Build history of the part. All positions in model axes, mm. Face numbers are marked on the shaded views. A direction names the side the tool comes from. Round coordinates to 2 decimals unless told otherwise and drop trailing zeros. Write each loop counter-clockwise with the first axis right and the second up, starting at its lowest first coordinate (ties: lowest second). Pieces come first, ordered by that corner, then holes. Notation, with made-up numbers: M 30,-36.75 L 82,-36.75 A28 cw 82,-15.75 Z; hole C 41,38.5 d8. An arc over 180 degrees is marked long. Use a Markdown table: item, result.
from build123d import *

# Parameters (mm, degrees)
EXTRUDE_3_DEPTH     = 5
SKETCH_1_R          = 9.79888
CUT_EXTRUDE_1_DEPTH = 1.65
SKETCH_1_9_R        = 3.15
SKETCH_3_8_R        = 1.65
SKETCH_3_9_R        = 1.648905
SKETCH_3_9_R_2      = 1.65
CUT_EXTRUDE_2_DEPTH = 5
EXTRUDE_4_DEPTH     = 28
SKETCH_10_R         = 11.19888
CUT_EXTRUDE_3_DEPTH = 3.35


with BuildPart() as part:
    # 草图7 → 凸台-拉伸3 (new body)
    with BuildSketch(Plane.XY):
        with BuildLine():
            Line((14, 14), (-14, 14))
            Line((-14, 14), (-14, 0))
            ThreePointArc((-14, 0), (-12.934313455, -5.357568053), (-9.899494937, -9.899494937))
            Line((-9.899494937, -9.899494937), (-2.121320344, -17.67766953))
            ThreePointArc((-2.121320344, -17.67766953), (0.000404905, -18.556181469), (2.121892965, -17.677096908))
            Line((2.121892965, -17.677096908), (9.899494937, -9.899494937))
            ThreePointArc((9.899494937, -9.899494937), (12.934313455, -5.357568053), (14, 0))
            Line((14, 0), (14, 14))
        make_face()
    extrude(amount=-EXTRUDE_3_DEPTH)

    # 草图1 → 切除-拉伸1 (cut)
    with BuildSketch(Plane.XY):
        Circle(SKETCH_1_R)
    extrude(amount=-CUT_EXTRUDE_1_DEPTH, mode=Mode.SUBTRACT)

    # 切除-放样1: read off the stored shape, not the designer's step
    # 切除-放样1 outline → 切除-放样1 (revolve, cut)
    with BuildSketch(Plane(origin=(10.6066, 10.606603436, 0), x_dir=(1, 0, 0), z_dir=(0, -1, 0))):
        Polygon((0, 0), (0, -1.5), (1.648905, -1.5), (3.15, 0), align=None)
    revolve(axis=Axis((10.6066, 10.606603436, 0), (0, 0, 1)), mode=Mode.SUBTRACT)

    # 切除-放样2: read off the stored shape, not the designer's step
    # 切除-放样2: loft between two sections, ruled curve by curve
    loft_2_from = [
        Edge.make_bspline([(-8.058196468, 12.45812698, 0), (-4.355149378, 7.361319916, 0), (-9.451956443, 3.658272826, 0), (-13.155003532, 8.755079891, 0), (-16.858050622, 13.851886955, 0), (-11.761243557, 17.554934045, 0), (-8.058196468, 12.45812698, 0)], [0, 0, 0, 0, 0.5, 0.5, 0.5, 1, 1, 1, 1], 3, [1, 0.333333333, 0.333333333, 1, 0.333333333, 0.333333333, 1]),
    ]
    loft_2_to = [
        Edge.make_bspline([(-9.518492924, 11.845518562, -1.5), (-7.040662671, 9.669304411, -1.5), (-9.216876823, 7.191474158, -1.5), (-11.694707076, 9.367688309, -1.5), (-14.172537329, 11.543902461, -1.5), (-11.996323177, 14.021732714, -1.5), (-9.518492924, 11.845518562, -1.5)], [0, 0, 0, 0, 0.5, 0.5, 0.5, 1, 1, 1, 1], 3, [1, 0.333333333, 0.333333333, 1, 0.333333333, 0.333333333, 1]),
    ]
    loft_2 = Solid(Shell([*[Face.make_surface_from_curves(loft_2_from[k], loft_2_to[k]) for k in range(1)], Face(Wire(loft_2_from)), Face(Wire(loft_2_to))]))
    add(loft_2, mode=Mode.SUBTRACT)

    # 草图1<9> → 切除-放样3 section 0
    with BuildSketch(Plane.XY):
        with Locations((0, -14.999996564)):
            Circle(SKETCH_1_9_R)
    # 草图3<8> → 切除-放样3 section 1
    with BuildSketch(Plane.XY.offset(-1.5)):
        with Locations((0, -14.999996564)):
            Circle(SKETCH_3_8_R)
    loft(mode=Mode.SUBTRACT)

    # 草图3<9> → 切除-拉伸2 (cut)
    with BuildSketch(Plane.XY.offset(-1.5)):
        with Locations(Location((-10.6066, 10.606603436, 0), (0, 0, 48.708))):
            Circle(SKETCH_3_9_R)
        with Locations((10.6066, 10.606603436)):
            Circle(SKETCH_3_9_R)
        with Locations((0, -14.999996564)):
            Circle(SKETCH_3_9_R_2)
    extrude(amount=-CUT_EXTRUDE_2_DEPTH, mode=Mode.SUBTRACT)

    # 草图9 → 凸台-拉伸4 (add)
    with BuildSketch(Plane(origin=(14, 0, 0), x_dir=(0, 0, -1), z_dir=(1, 0, 0))):
        Polygon((5, 14), (5, 16), (2, 16), (0, 14), align=None)
    extrude(amount=-EXTRUDE_4_DEPTH)

    # 草图10 → 切除-拉伸3 (cut)
    with BuildSketch(Plane(origin=(0, 0, -5), x_dir=(-1, 0, 0), z_dir=(0, 0, -1))):
        Circle(SKETCH_10_R)
    extrude(amount=-CUT_EXTRUDE_3_DEPTH, mode=Mode.SUBTRACT)


solid = part.part
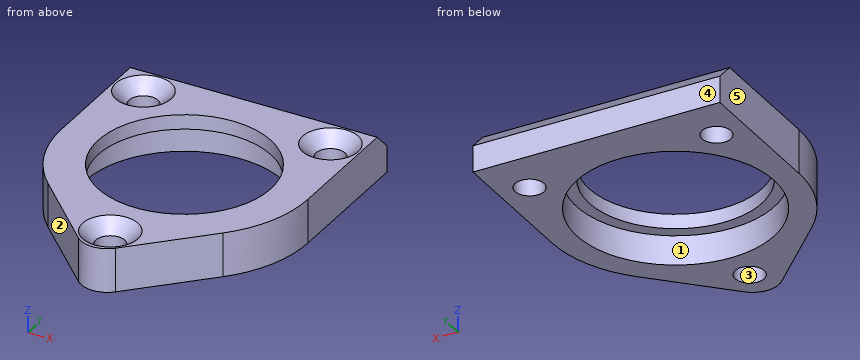
Q1. Two-plate mould, pull along Y, no slides. Class the marked faces 3, 4 and 5: +Y half, -Y half, draft (parallel to the pull), parting line (faces both ways), or undercut.
Response values:
| item | result |
|---|---|
| face 3 | undercut |
| face 4 | +Y half |
| face 5 | draft |
Q2. Drop flat-ended pins along their axis: P1, Ø3, axis at x = 0, y = -15, coming from the +Z side; P2, Ø1.5, axis at y = -12.5, z = -4.5, coming from the -X side. Give the stop position or say it passes through.
Response values:
| item | result |
|---|---|
| P1 | passes through |
| P2 | stops at x = -8.05 |
Q3. Cut at B-B on y = 6. Give the cut face in (x, z).
Response values:
| item | result |
|---|---|
| outline | M -14,-5 L -9.46,-5 L -9.46,-1.65 L -7.75,-1.65 L -7.75,0 L -14,0 Z; M 7.75,-1.65 L 9.46,-1.65 L 9.46,-5 L 14,-5 L 14,0 L 7.75,0 Z |
Q4. Cut at C-C on z = -3.5. Give the cut face in (x, y).
Response values:
| item | result |
|---|---|
| outline | M -14,0 A14 ccw -9.9,-9.9 L -2.12,-17.68 A3 ccw 2.12,-17.68 L 9.9,-9.9 A14 ccw 14,0 L 14,16 L -14,16 Z; hole C -10.61,10.61 d3.3; hole C 0,0 d22.4; hole C 0,-15 d3.3; hole C 10.61,10.61 d3.3 |
Q5. Cut at A-A on x = 0. Give the cut face in (y, z), and give its area (3 significant figures).
Response values:
| item | result |
|---|---|
| outline | M -18.56,-5 L -16.65,-5 L -16.65,-1.5 L -18.15,0 L -18.56,0 Z; M -13.35,-5 L -11.2,-5 L -11.2,-1.65 L -9.8,-1.65 L -9.8,0 L -11.85,0 L -13.35,-1.5 Z; M 9.8,-1.65 L 11.2,-1.65 L 11.2,-5 L 16,-5 L 16,-2 L 14,0 L 9.8,0 Z |
| area | 44.7 mm2 |
Q6. Cut at D-D on x = -4.75. Give the cut face in (y, z), and give its area (3 significant figures).
Response values:
| item | result |
|---|---|
| outline | M -15.05,-5 L -10.14,-5 L -10.14,-1.65 L -8.57,-1.65 L -8.57,0 L -15.05,0 Z; M 8.57,-1.65 L 10.14,-1.65 L 10.14,-5 L 16,-5 L 16,-2 L 14,0 L 8.57,0 Z |
| area | 57.0 mm2 |
Q7. Which spindle directions (+Z, -Z, +X, -X, +Y, -Y) get a long thin tool onto all of the face, cutting with end or side? Do the marked faces 1 and 2. Say none if no direction does.
Response values:
| item | result |
|---|---|
| face 1 | -Z |
| face 2 | +Z, -Z, -X, -Y |
Q8. Drill centre lines: L1, parallel to Y at x = 0, z = -3.15; L2, parallel to Y at x = 0, z = -1; L3, parallel to X at y = 10, z = -4.1. Where is each one in solid material? Low to high.
Response values:
| item | result |
|---|---|
| L1 | y = -18.56 to -16.65, -13.35 to -11.2, 11.2 to 16 |
| L2 | y = -18.56 to -17.15, -12.85 to -9.8, 9.8 to 15 |
| L3 | x = -14 to -12.14, -9.07 to -5.04, 5.04 to 9.07, 12.14 to 14 |
